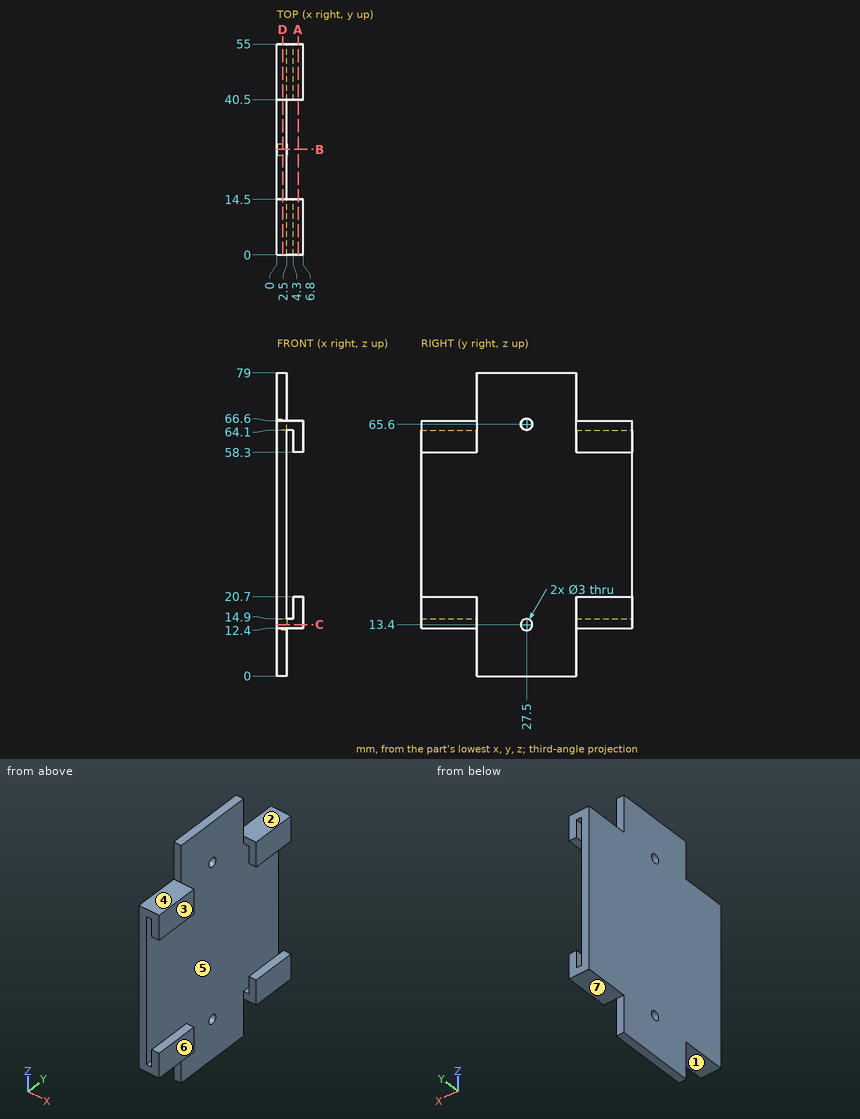
For this review, use the dimensioned drawing (mm, ordinates from the lowest corner) and the shaded views. A direction names the side the tool comes from. Round coordinates to 2 decimals unless told otherwise and drop trailing zeros. Write each loop counter-clockwise with the first axis right and the second up, starting at its lowest first coordinate (ties: lowest second). Pieces come first, ordered by that corner, then holes. Notation, with made-up numbers: (52, 16.25) -> (93, 16.25) arc R22 cw to (93, 44.25) -> close; hole circle Ø2 at (25, 28). An arc over 180 degrees is marked (long way). Use CSV: the item, a comma, the result in double quotes.
(1) Consider section D-D, the plane x = 1.5. Give the boundary of the cut face in (y, z), plus the area to 3 significant figures.
Computed values:
outline,"(0, 12.4) -> (14.5, 12.4) -> (14.5, 0) -> (40.5, 0) -> (40.5, 12.4) -> (55, 12.4) -> (55, 66.6) -> (40.5, 66.6) -> (40.5, 79) -> (14.5, 79) -> (14.5, 66.6) -> (0, 66.6) -> close; hole circle Ø3 at (27.5, 13.4); hole circle Ø3 at (27.5, 65.6)"
area,"3,610 mm²"
(2) For the marked faces 1, 2 and 3, list the 3-axis set-ups (+Z, -Z, +X, -X, +Y, -Y) from which the entire face can be reached by the end or side of a thin tool; tool diameter is ignored.
Computed values:
face 1,"-Z, +X, -X, -Y"
face 2,"+Z, +X, -X, +Y"
face 3,"+Z, -Z, +X, +Y, -Y"
(3) Consider section B-B, the plane y = 27.5. Give the boundary of the cut face in (x, z), plus the area to 4 significant figures.
Computed values:
outline,"(0, 0) -> (2.5, 0) -> (2.5, 11.9) -> (0, 11.9) -> close; (0, 14.9) -> (2.5, 14.9) -> (2.5, 64.1) -> (0, 64.1) -> close; (0, 67.1) -> (2.5, 67.1) -> (2.5, 79) -> (0, 79) -> close"
area,"182.5 mm²"
(4) Draft analysis for pull direction Z (two halves, no side actions). For the marked faces 4, 5, 6 and 7, state which applies: +Z half, -Z half, draft (parallel to the pull), parting line (faces both ways), or undercut.
Computed values:
face 4,"+Z half"
face 5,"undercut"
face 6,"draft"
face 7,"-Z half"
(5) To check wall thickness, follow L1, parallel to X at y = 5.5, z = 19; L2, parallel to Y at x = 1, z = 13.4; L3, parallel to Z at x = 1.25, y = 49.5. State the ranges of each line that lie inside material, in increasing order. Write a range as [from, to].
Computed values:
L1,"[0, 2.5], [4.3, 6.8]"
L2,"[0, 26], [29, 55]"
L3,"[12.4, 66.6]"
(6) Consider section A-A, the plane x = 5.5. Give the boundary of the cut face in (y, z), plus the area to 3 significant figures.
Computed values:
outline,"(0, 12.4) -> (14.5, 12.4) -> (14.5, 20.7) -> (0, 20.7) -> close; (0, 58.3) -> (14.5, 58.3) -> (14.5, 66.6) -> (0, 66.6) -> close; (40.5, 12.4) -> (55, 12.4) -> (55, 20.7) -> (40.5, 20.7) -> close; (40.5, 58.3) -> (55, 58.3) -> (55, 66.6) -> (40.5, 66.6) -> close"
area,"481 mm²"
(7) Consider section C-C, the plane z = 13.4. Give the boundary of the cut face in (x, y), plus the area to 3 significant figures.
Computed values:
outline,"(0, 0) -> (6.8, 0) -> (6.8, 14.5) -> (2.5, 14.5) -> (2.5, 26) -> (0, 26) -> close; (0, 29) -> (2.5, 29) -> (2.5, 40.5) -> (6.8, 40.5) -> (6.8, 55) -> (0, 55) -> close"
area,"255 mm²"
(8) Clearance check with flat-ended pins moving along their axes: P1, Ø2, axis at x = 1, z = 5.5, coming from the -Y side; P2, Ø2, axis at x = 1.5, z = 9, coming from the +Y side; P3, Ø2.5, axis at y = 27.5, z = 13.4, coming from the +X side; P4, Ø3, axis at x = 5, y = 10, coming from the -Z side. State where each tip first meets the part, or that it passes through.
Computed values:
P1,"y = 14.5"
P2,"y = 40.5"
P3,"through"
P4,"z = 12.4"
